Part model, mm, in its own coordinate system. Face numbers are marked on the shaded views. A direction names the side the tool comes from. Round coordinates to 2 decimals unless told otherwise and drop trailing zeros. Loops run counter-clockwise (first coordinate to the right, second up) from the corner with the lowest first, then second, coordinate; pieces in that order, holes last. Notation, with made-up numbers: (-30.75, 53) - (-12.75, 53) arc R26 ccw to (-12.75, 92) - close; hole circle Ø3 at (-19, -24.75). An arc over 180 degrees is marked (long way). Put each result on its own line as item: value.
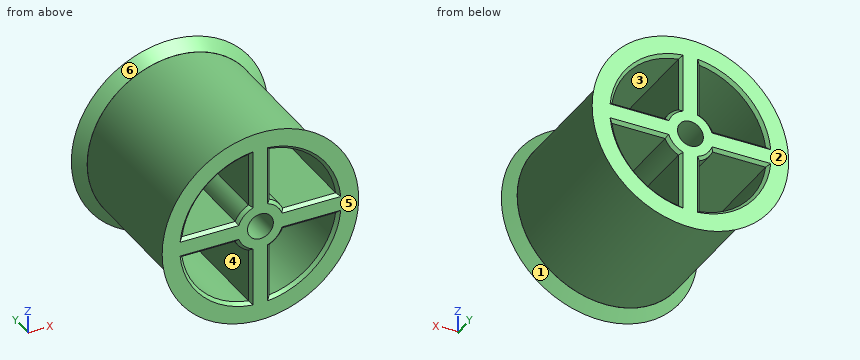
from build123d import *

# Parameters (mm, degrees)
F0_R     = 84.89324665
F1_DEPTH = 166
F2_R     = 95
F2_R_2   = 84.89324665
F3_DEPTH = 10
F4_R     = 95
F4_R_2   = 84.89324665
F5_DEPTH = 10
F6_SIZE  = 9.99999
F7_R     = 12.5
F8_DEPTH = 166.001
F9_SIZE  = 3


# Not quite as in the source:
# - a fillet or chamfer is up to 0.001 mm smaller than in the source, because OpenCascade refuses the exact size


with BuildPart() as f1:
    # F0 (on Front) → F1 (new body)
    with BuildSketch(Plane.XZ):
        Circle(F0_R)
    extrude(amount=F1_DEPTH)

    # F2 (on face) → F3 (join)
    with BuildSketch(Plane(origin=(0, 0, 0), x_dir=(-1, 0, 0), z_dir=(0, 1, 0))):
        Circle(F2_R)
        Circle(F2_R_2, mode=Mode.SUBTRACT)
    extrude(amount=-F3_DEPTH)

    # F4 (on face) → F5 (join)
    with BuildSketch(Plane.XZ.offset(166)):
        Circle(F4_R)
        Circle(F4_R_2, mode=Mode.SUBTRACT)
    extrude(amount=-F5_DEPTH)

    # F6 (size 10 in the source; OpenCascade refuses exactly that, so slightly less here)
    f6_edges = [f1.edges().sort_by_distance(p)[0] for p in [
        (95, -10, 0),
        (-95, -156, 0),
    ]]
    chamfer(f6_edges, length=F6_SIZE)

    # F7 (on face) → F8 (cut, through all)
    with BuildSketch(Plane(origin=(0, 0, 0), x_dir=(-1, 0, 0), z_dir=(0, 1, 0))):
        with BuildLine():
            Line((-10, 22.9128784748), (-10, 74.3303437366))
            ThreePointArc((-10, 74.3303437366), (-53.033008589, 53.033008589), (-74.3303437366, 10))
            Line((-74.3303437366, 10), (-22.9128784748, 10))
            ThreePointArc((-22.9128784748, 10), (-17.6776695297, 17.6776695297), (-10, 22.9128784748))
        make_face()
        with BuildLine():
            Line((22.9128784748, 10), (74.3303437366, 10))
            ThreePointArc((74.3303437366, 10), (53.033008589, 53.033008589), (10, 74.3303437366))
            Line((10, 74.3303437366), (10, 22.9128784748))
            ThreePointArc((10, 22.9128784748), (17.6776695297, 17.6776695297), (22.9128784748, 10))
        make_face()
        with BuildLine():
            ThreePointArc((-74.3303437366, -10), (-53.033008589, -53.033008589), (-10, -74.3303437366))
            Line((-10, -74.3303437366), (-10, -22.9128784748))
            ThreePointArc((-10, -22.9128784748), (-17.6776695297, -17.6776695297), (-22.9128784748, -10))
            Line((-22.9128784748, -10), (-74.3303437366, -10))
        make_face()
        with BuildLine():
            ThreePointArc((10, -74.3303437366), (53.033008589, -53.033008589), (74.3303437366, -10))
            Line((74.3303437366, -10), (22.9128784748, -10))
            ThreePointArc((22.9128784748, -10), (17.6776695297, -17.6776695297), (10, -22.9128784748))
            Line((10, -22.9128784748), (10, -74.3303437366))
        make_face()
        Circle(F7_R)
    extrude(amount=-F8_DEPTH, mode=Mode.SUBTRACT)

    # F9
    f9_edges = [f1.edges().sort_by_distance(p)[0] for p in [
        (-53.033009, -166, 53.033009),
        (-10, -166, 48.621611),
        (-48.621611, -166, 10),
        (-17.67767, -166, 17.67767),
        (53.033009, -166, 53.033009),
        (48.621611, -166, 10),
        (17.67767, -166, 17.67767),
        (10, -166, 48.621611),
        (48.621611, -166, -10),
        (53.033009, -166, -53.033009),
        (17.67767, -166, -17.67767),
        (10, -166, -48.621611),
        (-10, -166, -48.621611),
        (-17.67767, -166, -17.67767),
        (-48.621611, -166, -10),
        (-53.033009, -166, -53.033009),
        (-53.033009, 0, 53.033009),
        (-10, 0, 48.621611),
        (-17.67767, 0, 17.67767),
        (-48.621611, 0, 10),
        (-53.033009, 0, -53.033009),
        (-48.621611, 0, -10),
        (-17.67767, 0, -17.67767),
        (-10, 0, -48.621611),
        (10, 0, 48.621611),
        (53.033009, 0, 53.033009),
        (17.67767, 0, 17.67767),
        (48.621611, 0, 10),
        (17.67767, 0, -17.67767),
        (10, 0, -48.621611),
        (48.621611, 0, -10),
        (53.033009, 0, -53.033009),
    ]]
    chamfer(f9_edges, length=F9_SIZE)


solid = f1.part
1. Band-saw the part on C-C (y = -52.5). List the corners of the cut face in (x, z).
A:
outline: circle Ø169.79 at (0, 0); hole (-74.33, -10) arc R75 ccw to (-10, -74.33) - (-10, -22.91) arc R25 cw to (-22.91, -10) - close; hole (-74.33, 10) - (-22.91, 10) arc R25 cw to (-10, 22.91) - (-10, 74.33) arc R75 ccw to start; hole circle Ø25 at (0, 0); hole (10, -74.33) arc R75 ccw to (74.33, -10) - (22.91, -10) arc R25 cw to (10, -22.91) - close; hole (10, 22.91) arc R25 cw to (22.91, 10) - (74.33, 10) arc R75 ccw to (10, 74.33) - close
2. Tool access for the marked faces 4, 5 and 6: list every direction of +Z, -Z, +X, -X, +Y, -Y with a clear straight run to the whole face (end or side of a thin tool).
A:
face 4: +Y, -Y
face 5: +Z, -Z, +X, -X, -Y
face 6: none
3. Two-plate mould, pull along X, no slides. Class the marked faces 1, 2 and 3: pulls with the +X half, pulls with the -X half, needs draft (parallel to the pull), parting line crosses it, or undercut.
A:
face 1: parting line crosses it
face 2: needs draft
face 3: undercut
4. Band-saw the part on D-D (z = 38.5). Give the number of separate pieces and of enclosed holes in the cut face, plus the area to 3 significant figures.
A:
separate pieces: 3
enclosed holes: 0
area: 7,260 mm²
5. Pin check, flat tips, straight feed: P1, Ø15.5, axis at x = -49.5, y = -47.5, coming from the +Z side; P2, Ø2, axis at x = 59.5, z = -46.5, coming from the -Y side; P3, Ø1.5, axis at y = -101.5, z = -24.5, coming from the -X side. Stop position of each tip, or through.
A:
P1: stops at z = 73.92
P2: stops at y = -164.51
P3: stops at x = -81.5
6. Probe line 1 along Z through (x, y) = (0, -64); line 2 along X through (y, z) = (-88, -46.5); line 3 along Z through (x, y) = (18, -152). List the from-to ranges inside material, lowest first. Write a range as [from, to].
A:
line 1: z = [-84.89, -12.5], [12.5, 84.89]
line 2: x = [-71.03, -58.85], [-10, 10], [58.85, 71.03]
line 3: z = [-82.96, -72.81], [-17.35, 17.35], [72.81, 82.96]
